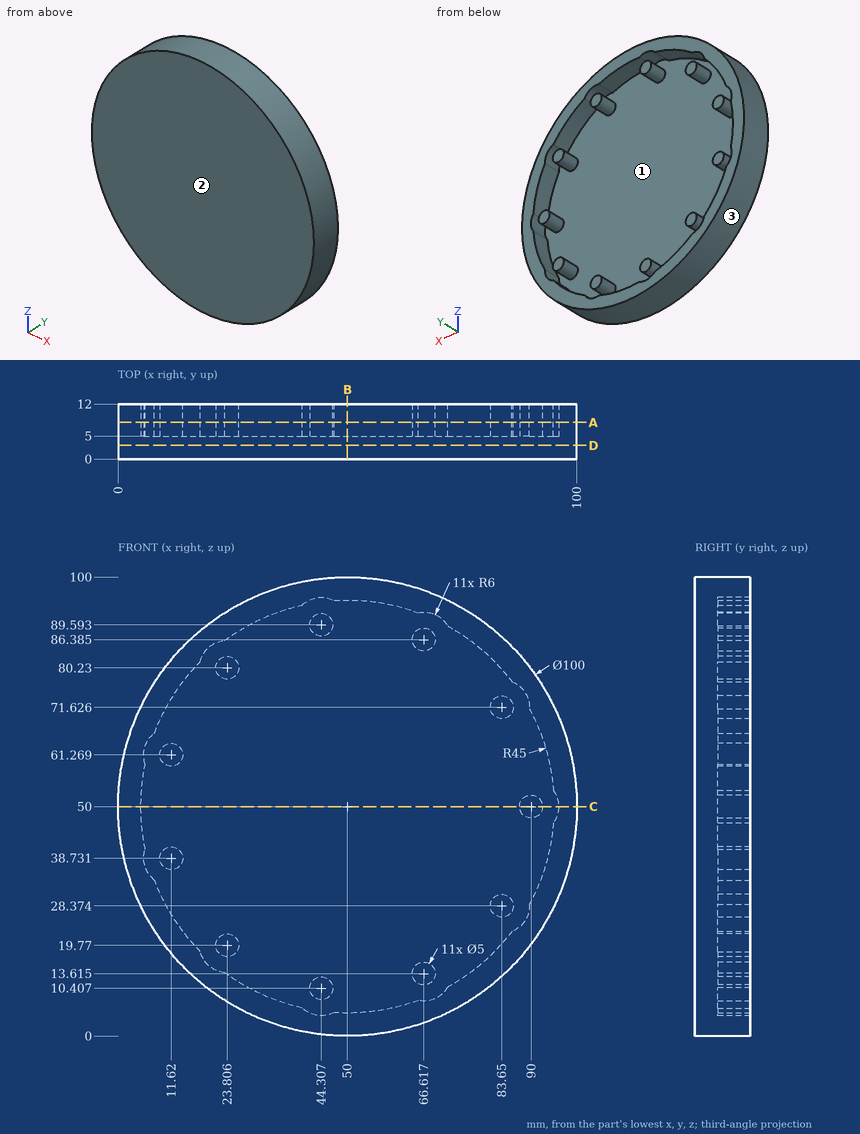
Print and shaded views of the part. All mm, measured from the part's lowest x, y and z. Round coordinates to 2 decimals unless told otherwise and drop trailing zeros. Order: outer loops, then holes, each group sorted by start corner. A loop starts at its lowest first (then second) coordinate and runs counter-clockwise, first axis right, second up. Notation, with made-up numbers: (58, 37) - (85, 37) arc R22 cw to (85, 60) - close; hole circle Ø4 at (9, 24). An arc over 180 degrees is marked (long way). Use a Markdown table: item, result.
1) Saw through at A-A on y = 8. Give the number of separate pieces and of enclosed holes in the cut face.
Recorded:
| item | result |
|---|---|
| separate pieces | 12 |
| enclosed holes | 1 |
2) Flat gauge pins, fed straight in: pin 1 Ø1.5 at (x, y) = (89.5, 5.5) entering from -Z; pin 2 Ø2 at (x, y) = (68, 9) entering from -Z; pin 3 Ø5 at (x, y) = (63, 4) entering from -Z (1 decimal). Where does each tip first touch, or does it go through?
Recorded:
| item | result |
|---|---|
| pin 1 | stops at z = 18.4 |
| pin 2 | stops at z = 2.98 |
| pin 3 | stops at z = 1.1 |
3) Wall check: L1, parallel to X at y = 5.5, z = 22 (1 decimal); L2, parallel to Y at x = 57, z = 61.5; L3, parallel to Z at x = 76, y = 9.5. Give the ranges that are in metal, low to high.
Recorded:
| item | result |
|---|---|
| L1 | x = 8.6 to 14.8, 22.7 to 24.9, 85.2 to 91.4 |
| L2 | y = 0 to 5 |
| L3 | z = 7.29 to 13.27, 86.73 to 92.71 |
4) Saw through at B-B on x = 50. Write the cut outline in (y, z).
Recorded:
| item | result |
|---|---|
| outline | (0, 0) - (12, 0) - (12, 5) - (5, 5) - (5, 95) - (12, 95) - (12, 100) - (0, 100) - close |
5) Saw through at C-C on z = 50. Write the cut outline in (x, y).
Recorded:
| item | result |
|---|---|
| outline | (0, 0) - (100, 0) - (100, 12) - (96, 12) - (96, 5) - (92.5, 5) - (92.5, 12) - (87.5, 12) - (87.5, 5) - (5, 5) - (5, 12) - (0, 12) - close |
6) Pull direction X, two halves, no side cores. Call the marked faces 1, 2 and 3: pulls with the +X half, pulls with the -X half, needs draft (parallel to the pull), parting line crosses it, or undercut.
Recorded:
| item | result |
|---|---|
| face 1 | undercut |
| face 2 | needs draft |
| face 3 | parting line crosses it |
7) Saw through at D-D on y = 3. Write the cut outline in (x, z).
Recorded:
| item | result |
|---|---|
| outline | circle Ø100 at (50, 50) |
